For this review, take the finished solid that the model builds, in its own axes (mm). A direction names the side the tool comes from. Coordinates: 2 decimals unless noted, no trailing zeros. Write each loop counter-clockwise with the first axis right and the second up, starting at its lowest first coordinate (ties: lowest second). Pieces come first, ordered by that corner, then holes.
1) We need section D-D on z = 2. Write out the cut boundary in (x, y) (3 decimals), then the cut area to 3 significant figures.
2) Mouldability with a two-part tool opening along X and no side actions: class faces 6 (the face through (2.3, 1.4, -1.3)), 7 (the face through (2.58, 0.99, -0.77)), 8 (the face through (-2.964, 0.764, -1.862)), 9 (the face through (1.45, 0, 0.63)) as pulls with the +X half, pulls with the -X half, needs draft (parallel to the pull), parting line crosses it, or undercut.
3) We need section B-B on x = 0. Write out the cut boundary in (y, z) (3 decimals).
4) We need section C-C on y = 4. Write out the cut boundary in (x, z) (3 decimals).
5) We need section A-A on z = 0. Write out the cut boundary in (x, y) (3 decimals), then the cut area to 3 significant figures.
6) For faces 1 (the face through (1.934, 0.37, -1.838)), 2 (the face through (-0.082, 3.722, 1.873)), 3 (the face through (3.09, 0.76, -1.64)), 4 (the face through (-0.625, 1, 3)), 5 (the face through (-2.266, 1.384, -1.318)), list the 3-axis set-ups (+Z, -Z, +X, -X, +Y, -Y) from which the entire face can be reached by the end or side of a thin tool; tool diameter is ignored.
7) Insertion check: P1, Ø0.5, axis at y = 1.5, z = 2.5, coming from the -X side (3 decimals); P2, Ø2, axis at x = -0.5, z = -1.5, coming from the -Y side; P3, Ø3, axis at x = -1, y = 5.5, coming from the -Z side (3 decimals); P4, Ø1.7, axis at x = 0, z = 0, coming from the +Y side. Each pin has a flat end and moves straight along its axis. Give the tip position at first contact, or say it passes through.
8) To check wall thickness, follow line 1 along X through (y, z) = (6, 0) (3 decimals); line 2 along X through (y, z) = (1.25, 0.95); line 3 along Z through (x, y) = (0.75, 7.25). State the ranges of each line that lie inside material, in increasing order.
from build123d import *

# Parameters (mm, degrees)
AUFSATZ_LINEAR_AUSTRAGEN1_DEPTH = 2
SCHNITT_LINEAR_AUSTRAGEN1_DEPTH = 4.5
KREISMUSTER1_COUNT              = 3


with BuildPart() as part:
    # Skizze1 → Rotation1 (revolve)
    with BuildSketch(Plane.XY, mode=Mode.PRIVATE) as rotation1_sk:
        Polygon((1.425, 0), (1.425, 8), (1.875, 7.55), (1.875, 0), align=None)
    revolve(rotation1_sk.sketch.rotate(Axis((0, 0, 0), (0, 1, 0)), 90), axis=Axis((0, 0, 0), (0, 1, 0)))  # turned: the seam where the file's is


with BuildPart() as body_2:
    # Skizze2 → Aufsatz-Linear austragen1 (new body)
    with BuildSketch(Plane(origin=(0, 0, 0), x_dir=(1, 0, 0), z_dir=(0, 1, 0))):
        with BuildLine():
            Line((-0.625, -3.443744328), (-0.625, -1.767766953))
            ThreePointArc((-0.625, -1.767766953), (0, -1.875), (0.625, -1.767766953))
            Line((0.625, -1.767766953), (0.625, -3.443744328))
            ThreePointArc((0.625, -3.443744328), (0, -3.5), (-0.625, -3.443744328))
        make_face()
    extrude(amount=AUFSATZ_LINEAR_AUSTRAGEN1_DEPTH)

    # Skizze3 → Schnitt-Linear austragen1 (cut, through all)
    with BuildSketch(Plane.XY):
        Polygon((-0.625, 2), (0.625, 0.75), (0.625, 2), align=None)
    extrude(amount=SCHNITT_LINEAR_AUSTRAGEN1_DEPTH, mode=Mode.SUBTRACT)


with BuildPart() as kreismuster1_1:
    # Kreismuster1: pattern copy
    add(body_2.part.rotate(Axis((0, 0, 0), (0, 1, 0)), 1 * 360 / KREISMUSTER1_COUNT))


with BuildPart() as kreismuster1_2:
    # Kreismuster1: pattern copy
    add(body_2.part.rotate(Axis((0, 0, 0), (0, 1, 0)), 2 * 360 / KREISMUSTER1_COUNT))


with BuildPart() as body_2_1:
    add(body_2.part)

    # Kombinieren1: union part, Kreismuster1_1, Kreismuster1_2
    add(part.part)
    add(kreismuster1_1.part)
    add(kreismuster1_2.part)


solid = body_2_1.part
Result:
1. outline: (-0.625, 0) - (0.625, 0) - (0.625, 0.75) - (-0.625, 2) - close
1. area: 1.72 mm2
2. face 6: undercut
2. face 7: pulls with the +X half
2. face 8: pulls with the -X half
2. face 9: needs draft
3. outline: (0, -1.875) - (7.55, -1.875) - (8, -1.425) - (0, -1.425) - close; (0, 1.425) - (8, 1.425) - (7.55, 1.875) - (1.375, 1.875) - (1.375, 3.5) - (0, 3.5) - close
4. outline: circle Ø3.75 at (0, 0); hole circle Ø2.85 at (0, 0)
5. outline: (-1.875, 0) - (-1.425, 0) - (-1.425, 8) - (-1.875, 7.55) - close; (1.425, 0) - (1.875, 0) - (1.875, 7.55) - (1.425, 8) - close
5. area: 7.00 mm2
6. face 1: -Z, +Y, -Y
6. face 2: +Y
6. face 3: -Z, +X, +Y, -Y
6. face 4: +Z, -X, +Y, -Y
6. face 5: -X, +Y
7. P1: stops at x = -0.625
7. P2: stops at y = 0
7. P3: stops at z = -1.875
7. P4: passes through
8. line 1: x = -1.875 to -1.425, 1.425 to 1.875
8. line 2: x = -1.62 to -1.06, 1.06 to 1.62
8. line 3: z = -1.72 to -1.21, 1.21 to 1.72
